Source: CAD feature listing. Evaluate the final solid. Frame: model axes, mm. Face numbers are marked on the shaded views. Coordinates: 2 decimals unless noted, no trailing zeros. Order: outer loops, then holes, each group sorted by start corner. A loop starts at its lowest first (then second) coordinate and runs counter-clockwise, first axis right, second up.
Item 1: Section A-A on z = 0. Return the cut outline in (x, y), then the cut area to 3 significant figures.
Item 2: Section B-B on y = 3.5. Return the cut outline in (x, z).
Item 3: Contact query for flat-ended pins moving along their axis: P1, Ø5, axis at y = 17.5, z = 23, coming from the +X side; P2, Ø2, axis at y = 4.5, z = -16.5, coming from the -X side; P3, Ø9.5, axis at y = 22.5, z = 24.99, coming from the -X side. Output: stop coordinate, or through.
Item 4: Section C-C on x = -14. Return the cut outline in (y, z), then the cut area to 3 significant figures.
Item 5: Mould query, pull axis Z, two halves, no side actions, for the marked faces 1, 2 and 3. Classes: released by +Z, released by -Z, zero draft, split by the parting line, or undercut.
Item 6: Section D-D on y = 7.5. Return the cut outline in (x, z).
Item 7: Ray query, line 1 (X direction, y = 22.5, z = 0); line 2 (Z direction, x = 9.5, y = 7.5); line 3 (Z direction, x = 7.5, y = 24). Return the intervals inside material, ascending.
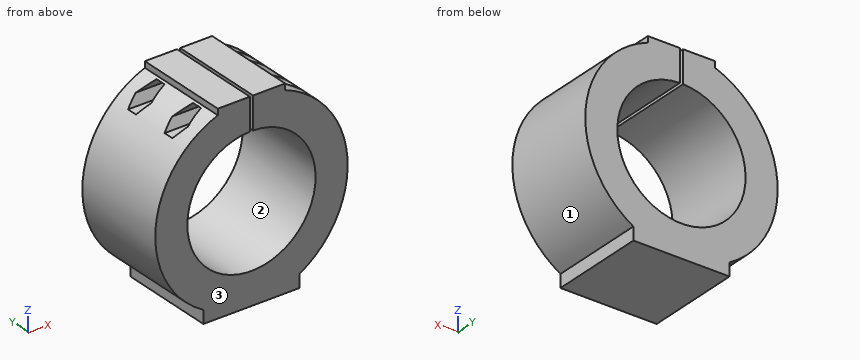
from build123d import *

# Parameters (mm, degrees)
BOSS_EXTRUDE1_DEPTH     = 30
CUT_EXTRUDE1_REACH      = 57
CUT_EXTRUDE1_END_RADIUS = 30
SKETCH7_R               = 3
CUT_EXTRUDE2_REACH      = 57
CUT_EXTRUDE2_END_RADIUS = 30
M3_CLEARANCE_HOLE1_D    = 3.4


with BuildPart() as part:
    # Sketch1 → Boss-Extrude1 (new body)
    with BuildSketch(Plane(origin=(0, 0, 0), x_dir=(1, 0, 0), z_dir=(0, 1, 0))):
        with BuildLine():
            Line((-0.5, -19.993749023), (-0.5, -29.993749023))
            Line((-0.5, -29.993749023), (-10.5, -29.993749023))
            Line((-10.5, -29.993749023), (-10.5, -28.102490993))
            ThreePointArc((-10.5, -28.102490993), (-29.896689894, -2.4875557), (-15, 25.980762114))
            Line((-15, 25.980762114), (-15, 30))
            Line((-15, 30), (15, 30))
            Line((15, 30), (15, 25.980762114))
            ThreePointArc((15, 25.980762114), (29.896689894, -2.4875557), (10.5, -28.102490993))
            Line((10.5, -28.102490993), (10.5, -29.993749023))
            Line((10.5, -29.993749023), (0.5, -29.993749023))
            Line((0.5, -29.993749023), (0.5, -19.993749023))
            ThreePointArc((0.5, -19.993749023), (0, 20), (-0.5, -19.993749023))
        make_face()
    extrude(amount=BOSS_EXTRUDE1_DEPTH)

    # Cut-Extrude1: up to this cylinder (the profile starts inside it)
    cut_extrude1_end = Plane(origin=(0, 15, 0), z_dir=(0, -1, 0)) * Cylinder(CUT_EXTRUDE1_END_RADIUS, 190, mode=Mode.PRIVATE)
    # Sketch7 → Cut-Extrude1 (cut, up to the surface)
    with BuildSketch(Plane(origin=(5, 0, 0), x_dir=(0, 0, -1), z_dir=(1, 0, 0)), mode=Mode.PRIVATE) as cut_extrude1_sk1:
        with Locations(Location((-24.993749023, 22.5, 0), (0, 0, 180))):
            Circle(SKETCH7_R)
    cut_extrude1_tool1 = extrude(cut_extrude1_sk1.sketch, amount=CUT_EXTRUDE1_REACH, mode=Mode.PRIVATE) & cut_extrude1_end
    add(cut_extrude1_tool1.solids().sort_by_distance((5, 22.5, 24.993749))[0], mode=Mode.SUBTRACT)
    # Sketch7 → Cut-Extrude1 (cut, up to the surface)
    with BuildSketch(Plane(origin=(5, 0, 0), x_dir=(0, 0, -1), z_dir=(1, 0, 0)), mode=Mode.PRIVATE) as cut_extrude1_sk2:
        with Locations(Location((-24.993749023, 7.5, 0), (0, 0, 180))):
            Circle(SKETCH7_R)
    cut_extrude1_tool2 = extrude(cut_extrude1_sk2.sketch, amount=CUT_EXTRUDE1_REACH, mode=Mode.PRIVATE) & cut_extrude1_end
    add(cut_extrude1_tool2.solids().sort_by_distance((5, 7.5, 24.993749))[0], mode=Mode.SUBTRACT)

    # Cut-Extrude2: up to this cylinder (the profile starts inside it)
    cut_extrude2_end = Plane(origin=(0, 15, 0), z_dir=(0, -1, 0)) * Cylinder(CUT_EXTRUDE2_END_RADIUS, 190, mode=Mode.PRIVATE)
    # Sketch8 → Cut-Extrude2 (cut, up to the surface)
    with BuildSketch(Plane(origin=(-5, 0, 0), x_dir=(0, 0, -1), z_dir=(1, 0, 0)), mode=Mode.PRIVATE) as cut_extrude2_sk1:
        Polygon((-24.993749023, 19.266838493), (-22.193749023, 20.883419246), (-22.193749023, 24.116580754), (-24.993749023, 25.733161507), (-27.793749023, 24.116580754), (-27.793749023, 20.883419246), align=None)
    cut_extrude2_tool1 = extrude(cut_extrude2_sk1.sketch, amount=-CUT_EXTRUDE2_REACH, mode=Mode.PRIVATE) & cut_extrude2_end
    add(cut_extrude2_tool1.solids().sort_by_distance((-5, 22.5, 24.993749))[0], mode=Mode.SUBTRACT)
    # Sketch8 → Cut-Extrude2 (cut, up to the surface)
    with BuildSketch(Plane(origin=(-5, 0, 0), x_dir=(0, 0, -1), z_dir=(1, 0, 0)), mode=Mode.PRIVATE) as cut_extrude2_sk2:
        Polygon((-24.993749023, 4.266838493), (-22.193749023, 5.883419246), (-22.193749023, 9.116580754), (-24.993749023, 10.733161507), (-27.793749023, 9.116580754), (-27.793749023, 5.883419246), align=None)
    cut_extrude2_tool2 = extrude(cut_extrude2_sk2.sketch, amount=-CUT_EXTRUDE2_REACH, mode=Mode.PRIVATE) & cut_extrude2_end
    add(cut_extrude2_tool2.solids().sort_by_distance((-5, 7.5, 24.993749))[0], mode=Mode.SUBTRACT)

    # M3 Clearance Hole1 (through all)
    with Locations(Plane(origin=(5, 0, 0), x_dir=(0, 0, -1), z_dir=(1, 0, 0))):
        with Locations((-24.993749023, 7.5), (-24.993749023, 22.5)):
            Hole(M3_CLEARANCE_HOLE1_D / 2)


solid = part.part
Answer list:
1. outline: (-30, 0) - (-20, 0) - (-20, 30) - (-30, 30) - close; (20, 0) - (30, 0) - (30, 30) - (20, 30) - close
1. area: 600 mm2
2. outline: (-15, -30) - (15, -30) - (15, -25.98) arc R30 ccw to (10.5, 28.1) - (10.5, 29.99) - (0.5, 29.99) - (0.5, 19.99) arc R20 cw (long way) to (-0.5, 19.99) - (-0.5, 29.99) - (-10.5, 29.99) - (-10.5, 28.1) arc R30 ccw to (-15, -25.98) - close
3. P1: stops at x = 21.9
3. P2: stops at x = -25.69
3. P3: stops at x = -22.14
4. outline: (0, -30) - (30, -30) - (30, -14.28) - (0, -14.28) - close; (0, 14.28) - (30, 14.28) - (30, 26.53) - (24.84, 26.53) - (25.73, 24.99) - (24.12, 22.19) - (20.88, 22.19) - (19.27, 24.99) - (20.16, 26.53) - (9.84, 26.53) - (10.73, 24.99) - (9.12, 22.19) - (5.88, 22.19) - (4.27, 24.99) - (5.16, 26.53) - (0, 26.53) - close
4. area: 795 mm2
5. face 1: split by the parting line
5. face 2: undercut
5. face 3: zero draft
6. outline: (-20.19, 22.19) arc R30 ccw to (-15, -25.98) - (-15, -30) - (15, -30) - (15, -25.98) arc R30 ccw to (20.4, 21.99) - (5, 21.99) - (5, 23.29) - (0.5, 23.29) - (0.5, 19.99) arc R20 cw (long way) to (-0.5, 19.99) - (-0.5, 23.29) - (-5, 23.29) - (-5, 22.19) - close; (-11.29, 27.79) - (-5, 27.79) - (-5, 26.69) - (-0.5, 26.69) - (-0.5, 29.99) - (-10.5, 29.99) - (-10.5, 28.1) arc R30 ccw to start; (0.5, 26.69) - (5, 26.69) - (5, 27.99) - (10.79, 27.99) arc R30 ccw to (10.5, 28.1) - (10.5, 29.99) - (0.5, 29.99) - close
7. line 1: x = -30 to -20, 20 to 30
7. line 2: z = -30 to -17.6, 17.6 to 21.99, 27.99 to 29.99
7. line 3: z = -30 to -18.54, 18.54 to 22.4, 27.59 to 29.99
